The drawing under review shows one solid part. Ordinate dimensions are in mm from its lowest x, y, z. Coordinates: 2 decimals unless noted, no trailing zeros. Order: outer loops, then holes, each group sorted by start corner. A loop starts at its lowest first (then second) coordinate and runs counter-clockwise, first axis right, second up.
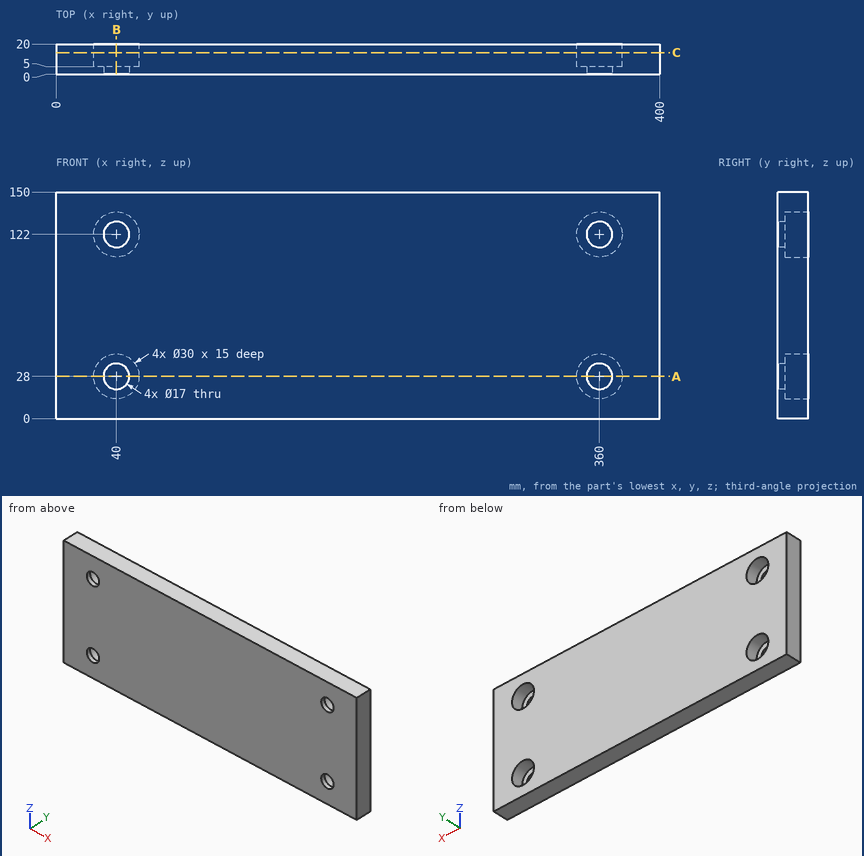
(1) Consider section C-C (y = 14.25). Give the boundary of the cut face in (x, z), then the cut area to 3 significant figures.
(2) Consider section A-A (z = 28). Give the boundary of the cut face in (x, y), then the cut area to 3 significant figures.
(3) Wall thickness on line 1 (X direction, y = 16, z = 122); line 2 (Z direction, x = 360, y = 1.3); line 3 (Z direction, x = 360, y = 14.25): over which ranges is each line inside the solid? List them lowest first.
(4) Insertion check: pin 1 Ø15 at (x, z) = (359.5, 125.5) entering from +Y; pin 2 Ø15.5 at (x, z) = (360, 122) entering from -Y. Each pin has a flat end and moves straight along its axis. Give the tip position at first contact, or say it passes through.
(5) Consider section B-B (x = 40). Give the boundary of the cut face in (y, z).
Findings:
1. outline: (0, 0) - (400, 0) - (400, 150) - (0, 150) - close; hole circle Ø30 at (40, 28); hole circle Ø30 at (40, 122); hole circle Ø30 at (360, 28); hole circle Ø30 at (360, 122)
1. area: 57,200 mm2
2. outline: (0, 0) - (31.5, 0) - (31.5, 5) - (25, 5) - (25, 20) - (0, 20) - close; (48.5, 0) - (351.5, 0) - (351.5, 5) - (345, 5) - (345, 20) - (55, 20) - (55, 5) - (48.5, 5) - close; (368.5, 0) - (400, 0) - (400, 20) - (375, 20) - (375, 5) - (368.5, 5) - close
2. area: 6,930 mm2
3. line 1: x = 0 to 25, 55 to 345, 375 to 400
3. line 2: z = 0 to 19.5, 36.5 to 113.5, 130.5 to 150
3. line 3: z = 0 to 13, 43 to 107, 137 to 150
4. pin 1: stops at y = 5
4. pin 2: passes through
5. outline: (0, 0) - (20, 0) - (20, 13) - (5, 13) - (5, 19.5) - (0, 19.5) - close; (0, 36.5) - (5, 36.5) - (5, 43) - (20, 43) - (20, 107) - (5, 107) - (5, 113.5) - (0, 113.5) - close; (0, 130.5) - (5, 130.5) - (5, 137) - (20, 137) - (20, 150) - (0, 150) - close
